For this review, take the finished solid that the model builds, in its own axes (mm). A direction names the side the tool comes from. Round coordinates to 2 decimals unless told otherwise and drop trailing zeros. Write each loop counter-clockwise with the first axis right and the second up, starting at its lowest first coordinate (ties: lowest second). Pieces come first, ordered by that corner, then holes. Notation, with made-up numbers: (-6.5, 14) -> (49.5, 14) arc R29 ccw to (49.5, 50) -> close; hole circle Ø9 at (13.25, 82.25). An arc over 180 degrees is marked (long way). Write each question's results on one line, items separated by ' | '. Start each with the question number.
Item 1: To check wall thickness, follow line 1 along Z through (x, y) = (50, 3.15); line 2 along X through (y, z) = (-16.75, -2.5); line 3 along Y through (x, z) = (51, 4.25). State the ranges of each line that lie inside material, in increasing order.
Item 2: Add section D-D (x = 2). State the section outline as (y, z) points, plus the area to 3 significant figures.
Item 3: Clearance check with flat-ended pins moving along their axes: pin 1 (2.5 mm diameter, centred on y = -4, z = 2, fed in from +X); pin 2 (6 mm diameter, centred on x = 5, y = -11, fed in from +Z); pin 3 (5.5 mm diameter, centred on x = 0, z = 0, fed in from -Y); pin 4 (5 mm diameter, centred on x = -2, z = 0, fed in from -Y). State where each tip first meets the part, or that it passes through.
Item 4: Add section B-B (z = 1.25). State the section outline as (x, y) points, plus the area to 3 significant figures.
Item 5: Tool access review of faces 1 (the flat face through (25, -7, 0)), 2 (the flat face through (46.8, 0, -0.1)), 3 (the flat face through (3, 0, -1)): name each direction out of +Z, -Z, +X, -X, +Y, -Y from which nothing blocks a thin tool from reaching the whole face with its end or side.
Item 6: The part is to be moulded in two halves that separate along X. For faces 4 (the flat face through (25, -7, -5)), 5 (the flat face through (44, 2, 0)), 6 (the flat face through (33.75, -8, 3)), 7 (the flat face through (43.75, -10, -3)), say which applies: +X half, -X half, draft (parallel to the pull), parting line (faces both ways), or undercut.
Item 7: Add section C-C (y = 3.25). State the section outline as (x, z) points, plus the area to 3 significant figures.
Item 8: Add section A-A (y = -17.5). State the section outline as (x, z) points.
Autodesk Fusion 360 part; units mm, degrees
sketch "Sketch1" plane through (0, 0, 0) normal (0, 1, 0) x (1, 0, 0)
  circle A0 centre (0, 0) radius 2.95
  line L0 (0, 0) -> (25, 0) construction
  line L1 (25, -32.2093) -> (25, 32.2093)
  circle A1 centre (0, 0) radius 5
  line L2 (0, 5) -> (25, 5)
  line L3 (5, 0) -> (25, 0)
  line L4 (16.25, 0) -> (16.25, -5)
  line L5 (16.25, -5) -> (11.25, -5)
  line L6 (11.25, -5) -> (6.25, 0)
  line L7 (11.25, -5) -> (18.3211, -5) construction
  dimension "d1" = 5.9
  dimension "d2" = 25
  dimension "d3" = 10
  dimension "d4" = 17.5
  dimension "d5" = 5
  dimension "d6" = 5
  dimension "d7" = 135
extrude "Extrude1" add sketch "Sketch1" along normal blind 5
sketch "Sketch2" plane through (0, 0, 0) normal (0, -1, 0) x (1, 0, 0)
  circle A0 centre (0, 0) radius 2.95
  line L0 (25, 0) -> (16.25, 0)
  line L1 (16.25, 0) -> (16.25, 5)
  line L2 (16.25, 5) -> (11.25, 5)
  line L3 (11.25, 5) -> (6.25, 0)
  line L4 (6.25, 0) -> (5, 0)
  arc A1 (5, 0) -> (0, -5) centre (0, 0) ccw
  line L5 (0, -5) -> (25, -5)
  line L6 (25, -5) -> (25, 0)
  line L7 (6.25, 0) -> (6.25, -5)
extrude "Extrude2" add sketch "Sketch2" along normal blind 20 contours L0 L1 L2 L3 L5 L6 L7
sketch "Sketch3" plane through (0, -20, 0) normal (0, -1, 0) x (1, 0, 0)
  line L0 (6.25, 0) -> (6.25, -5)
  line L1 (6.25, -5) -> (25, -5)
  line L2 (25, -5) -> (25, 0)
  line L3 (25, 0) -> (16.25, 0)
  line L4 (16.25, 0) -> (16.25, 5)
  line L5 (16.25, 5) -> (11.25, 5)
  line L6 (11.25, 5) -> (6.25, 0)
  line L7 (6.25, -5) -> (6.25, 0)
  line L8 (6.25, 0) -> (5, 0)
  arc A0 (5, 0) -> (0, -5) centre (0, 0) ccw
  line L9 (0, -5) -> (6.25, -5)
  circle A1 centre (0, 0) radius 2.95
extrude "Extrude3" add sketch "Sketch3" along normal blind 5
mirror "Mirror1" about plane through (25, 0, -5) normal (1, 0, 0) of bodies 1 merged
sketch "Sketch4" plane through (0, 0, 0) normal (0, 0, 1) x (-1, 0, 0)
  line L0 (-33.75, -5) -> (-16.25, -5)
  line L1 (-16.25, -5) -> (-16.25, 25)
  line L2 (-16.25, 25) -> (-33.75, 25)
  line L3 (-33.75, 25) -> (-33.75, -5)
  line L4 (-33.75, 25) -> (-16.25, 25)
  line L5 (-16.25, 25) -> (-16.25, 20)
  line L6 (-16.25, 20) -> (-33.75, 20)
  line L7 (-33.75, 20) -> (-33.75, 25)
  dimension "d16" = 17.5
  dimension "d17" = 5
extrude "Extrude4" cut sketch "Sketch4" against normal blind 5 contours L1 L2 L3 L4 L5 L6 L7
extrude "Extrude5" cut 2 faces at (11.25, -25, 0) (38.75, -25, 0) along direction (0, 1, 0) blind 5
Responses:
1) line 1: z = -5 to -2.95, 2.95 to 5 | line 2: x = 6.25 to 43.75 | line 3: y = 0 to 5
2) outline: (0, -5) -> (5, -5) -> (5, -2.17) -> (0, -2.17) -> close; (0, 2.17) -> (5, 2.17) -> (5, 4.58) -> (0, 4.58) -> close | area: 26.2 mm^2
3) pin 1: stops at x = 43 | pin 2: stops at z = 1.75 | pin 3: passes through | pin 4: stops at y = 0
4) outline: (-4.84, 0) -> (-2.67, 0) -> (-2.67, 5) -> (-4.84, 5) -> close; (2.67, 0) -> (4.84, 0) -> (4.84, 5) -> (2.67, 5) -> close; (7.5, -20) -> (16.25, -20) -> (16.25, 5) -> (7.5, 5) -> close; (33.75, -20) -> (42.5, -20) -> (42.5, 5) -> (33.75, 5) -> close; (45.16, 0) -> (47.33, 0) -> (47.33, 5) -> (45.16, 5) -> close; (52.67, 0) -> (54.84, 0) -> (54.84, 5) -> (52.67, 5) -> close | area: 481 mm^2
5) face 1: +Z, +Y, -Y | face 2: +Z, -Z, +X, -Y | face 3: +Z, -Z, -X, -Y
6) face 4: draft | face 5: undercut | face 6: undercut | face 7: +X half
7) outline: (0, -5) -> (50, -5) arc R5 ccw (long way) to (45, 0) -> (43.75, 0) -> (38.75, 5) -> (33.75, 5) -> (33.75, 0) -> (16.25, 0) -> (16.25, 5) -> (11.25, 5) -> (6.25, 0) -> (5, 0) arc R5 ccw (long way) to start; hole circle Ø5.9 at (0, 0); hole circle Ø5.9 at (50, 0) | area: 388 mm^2
8) outline: (6.25, -5) -> (43.75, -5) -> (43.75, 0) -> (38.75, 5) -> (33.75, 5) -> (33.75, 0) -> (16.25, 0) -> (16.25, 5) -> (11.25, 5) -> (6.25, 0) -> close
